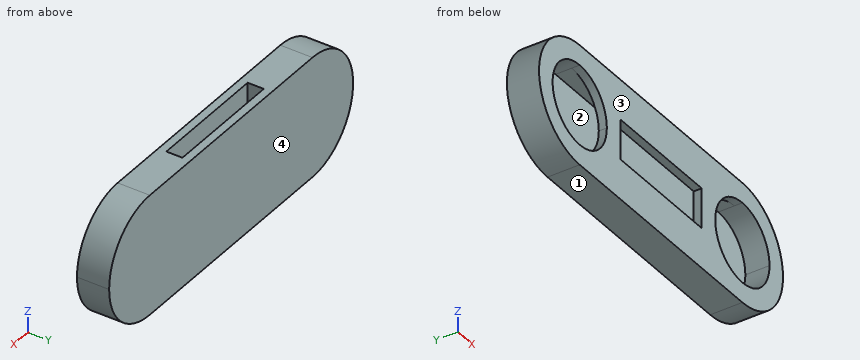
from build123d import *

# Parameters (mm, degrees)
F0_W      = 152.4
F0_H      = 76.2
F1_DEPTH  = 20.32
F2_W      = 76.2
F2_H      = 10.16
F3_DEPTH  = 63.5
F5_W      = 10.16
F5_H      = 50.8
F6_DEPTH  = 152.4
F7_DEPTH  = 20.32
F9_DEPTH  = 15.24
F10_W     = 76.2
F10_H     = 25.4
F11_DEPTH = 5.08


with BuildPart() as f1:
    # F0 (on Front) → F1 (new body)
    with BuildSketch(Plane.XZ):
        with Locations((28.4777595112, -5.5712945759)):
            Rectangle(F0_W, F0_H)
    extrude(amount=F1_DEPTH)

    # F2 (on face) → F3 (cut)
    with BuildSketch(Plane.XY.offset(32.5287054241)):
        with Locations((28.4777595112, -10.16)):
            Rectangle(F2_W, F2_H)
    extrude(amount=-F3_DEPTH, mode=Mode.SUBTRACT)

    # F5 (on face) → F6 (cut)
    with BuildSketch(Plane(origin=(-47.7222404888, 0, 0), x_dir=(0, -1, 0), z_dir=(-1, 0, 0))):
        with Locations((10.16, -5.5712945759)):
            Rectangle(F5_W, F5_H)
    extrude(amount=-F6_DEPTH, mode=Mode.SUBTRACT)

    # F4 (on face) → F7 (join)
    with BuildSketch(Plane.XZ.offset(20.32)):
        with BuildLine():
            Line((-47.7222404888, -43.6712945759), (-47.7222404888, 32.5287054241))
            ThreePointArc((-47.7222404888, 32.5287054241), (-85.8222404888, -5.5712945759), (-47.7222404888, -43.6712945759))
        make_face()
        with BuildLine():
            ThreePointArc((142.7777595112, -5.5712945759), (131.6185278744, 21.3694737873), (104.6777595112, 32.5287054241))
            Line((104.6777595112, 32.5287054241), (104.6777595112, -43.6712945759))
            ThreePointArc((104.6777595112, -43.6712945759), (131.6185278744, -32.5120629391), (142.7777595112, -5.5712945759))
        make_face()
    extrude(amount=-F7_DEPTH)

    # F8 (on face) → F9 (cut)
    with BuildSketch(Plane.XZ.offset(20.32)):
        with BuildLine():
            Line((-47.7222404888, -30.9712945759), (-47.7222404888, 19.8287054241))
            ThreePointArc((-47.7222404888, 19.8287054241), (-73.1222404888, -5.5712945759), (-47.7222404888, -30.9712945759))
        make_face()
        with BuildLine():
            ThreePointArc((-22.3222404888, -5.5712945759), (-29.7617282466, 12.3892176662), (-47.7222404888, 19.8287054241))
            Line((-47.7222404888, 19.8287054241), (-47.7222404888, -30.9712945759))
            ThreePointArc((-47.7222404888, -30.9712945759), (-29.7617282466, -23.5318068181), (-22.3222404888, -5.5712945759))
        make_face()
        with BuildLine():
            Line((104.6777595112, -30.9712945759), (104.6777595112, 19.8287054241))
            ThreePointArc((104.6777595112, 19.8287054241), (79.2777595112, -5.5712945759), (104.6777595112, -30.9712945759))
        make_face()
        with BuildLine():
            ThreePointArc((130.0777595112, -5.5712945759), (122.6382717534, 12.3892176662), (104.6777595112, 19.8287054241))
            Line((104.6777595112, 19.8287054241), (104.6777595112, -30.9712945759))
            ThreePointArc((104.6777595112, -30.9712945759), (122.6382717534, -23.5318068181), (130.0777595112, -5.5712945759))
        make_face()
    extrude(amount=-F9_DEPTH, mode=Mode.SUBTRACT)

    # F10 (on face) → F11 (cut)
    with BuildSketch(Plane.XZ.offset(20.32)):
        with Locations((28.4777595112, -5.5712945759)):
            Rectangle(F10_W, F10_H)
    extrude(amount=-F11_DEPTH, mode=Mode.SUBTRACT)


solid = f1.part
Input: part model. Units: mm. Frame: model coordinates. Face numbers are marked on the shaded views. Give positions to 0.01 mm unless a question says otherwise; leave off trailing zeros. Order: outer loops, then holes, each group sorted by start corner. A loop starts at its lowest first (then second) coordinate and runs counter-clockwise, first axis right, second up. Notation, with made-up numbers: M 88,29 L 114,29 A22 ccw 114,61 Z; hole C -4.5,-14.5 d6. An arc over 180 degrees is marked long. Answer as a JSON object with one key per item and string values.
1. Ray query, line 1 (X direction, y = -15.5, z = 12); line 2 (Y direction, x = -19.5, z = 11.5); line 3 (Z direction, x = 23, y = -16). Return the intervals inside material, ascending. Write a range as [from, to].
Result sheet:
{"line 1": "[-81.53, -66.06], [-29.38, 86.34], [123.02, 138.48]", "line 2": "[-20.32, -15.24], [-5.08, 0]", "line 3": "[-43.67, -18.27], [7.13, 32.53]"}
2. Cut plane A-A, the plane x = 21.5. Output: boundary loops of the cut face in (y, z), and give its area (3 significant figures).
Result sheet:
{"outline": "M -20.32,-43.67 L 0,-43.67 L 0,32.53 L -5.08,32.53 L -5.08,-30.97 L -15.24,-30.97 L -15.24,-18.27 L -20.32,-18.27 Z; M -20.32,7.13 L -15.24,7.13 L -15.24,32.53 L -20.32,32.53 Z", "area": "774 mm²"}
3. Cut plane B-B, the plane z = -10.5. Output: boundary loops of the cut face in (x, y), and give its area (3 significant figures).
Result sheet:
{"outline": "M -85.5,-20.32 L -72.64,-20.32 L -72.64,-5.08 L 129.59,-5.08 L 129.59,-20.32 L 142.46,-20.32 L 142.46,0 L -85.5,0 Z; M -22.81,-20.32 L -9.62,-20.32 L -9.62,-15.24 L -22.81,-15.24 Z; M 66.58,-20.32 L 79.76,-20.32 L 79.76,-15.24 L 66.58,-15.24 Z", "area": "1,680 mm²"}
4. Cut plane C-C, the plane y = -10.75. Output: boundary loops of the cut face in (x, z), and give its area (3 significant figures).
Result sheet:
{"outline": "M -47.72,-43.67 L 104.68,-43.67 A38.1 ccw 104.68,32.53 L 66.58,32.53 L 66.58,19.83 L 104.68,19.83 A25.4 cw 104.68,-30.97 L -47.72,-30.97 A25.4 cw -47.72,19.83 L -9.62,19.83 L -9.62,32.53 L -47.72,32.53 A38.1 ccw Z", "area": "5,440 mm²"}
5. Cut plane D-D, the plane z = 14.5. Output: boundary loops of the cut face in (x, y), and give its area (3 significant figures).
Result sheet:
{"outline": "M -80.11,-20.32 L -63.29,-20.32 L -63.29,-5.08 L 120.24,-5.08 L 120.24,-20.32 L 137.06,-20.32 L 137.06,0 L -80.11,0 Z; M -32.16,-20.32 L 89.11,-20.32 L 89.11,-15.24 L -32.16,-15.24 Z", "area": "2,230 mm²"}
6. First-contact query: P1, Ø5, axis at x = 54, y = -8.5, coming from the +Z side; P2, Ø3, axis at y = -11.5, z = 28.5, coming from the +X side; P3, Ø1.5, axis at y = -16.5, z = -3.5, coming from the +X side. Flat tips, straight axial feed; report the tip coordinate or a pass-through.
Result sheet:
{"P1": "z = -30.97", "P2": "x = 124.44", "P3": "x = 142.75"}
7. Pull-direction query (Y, two-part tool) for the marked faces 1, 2, 3 and 4; classes: +Y half, -Y half, draft (parallel to the pull), parting line (faces both ways), or undercut.
Result sheet:
{"face 1": "draft", "face 2": "undercut", "face 3": "-Y half", "face 4": "+Y half"}
